Input: part model. Units: mm. Frame: model coordinates. Coordinates: 2 decimals unless noted, no trailing zeros. Loops run counter-clockwise (first coordinate to the right, second up) from the corner with the lowest first, then second, coordinate; pieces in that order, holes last. Notation, with made-up numbers: M -14,47 L 2,47 A10 ccw 2,55 Z; hole C 1.25,61 d10. An arc over 180 degrees is marked long. Use a Markdown table: item, result. Add a question column.
1. Section C-C on y = 2.25. Output: boundary loops of the cut face in (x, z), then the cut area to 3 significant figures.
2. Line query: L1, parallel to Y at x = 1, z = -2; L2, parallel to Z at x = 4.5, y = -1; L3, parallel to Z at x = 2.25, y = -2. Output: solid intervals per line, ascending. Write a range as [from, to].
3. Section B-B on x = 2.5. Output: boundary loops of the cut face in (y, z) (3 decimals), then the cut area to 3 significant figures.
4. Section A-A on z = 12. Output: boundary loops of the cut face in (x, y), then the cut area to 3 significant figures.
5. Pin query (flat end, axial travel): pin 1 (2 mm diameter, centred on x = 0.5, y = -4.5, fed in from +Z); pin 2 (1.8 mm diameter, centred on y = 0, z = -12, fed in from -X); pin 3 (0.7 mm diameter, centred on y = 0, z = 15, fed in from +X); pin 4 (2 mm diameter, centred on x = 5.5, y = 3, fed in from -Z). Return the tip coordinate at first contact, or that it passes through.
6. Section D-D on y = 6.5. Output: boundary loops of the cut face in (x, z).
7. Draft query along Y for faces 1 (the cylindrical face through (3.131, -0.119, -14.463)), 2 (the flat face through (3, -8, 0)), 3 (the cylindrical face through (3, 0, -26)), 4 (the flat face through (6.35, 3.4, 0.4)). Return one class per face: +Y half, -Y half, draft (parallel to the pull), parting line (faces both ways), or undercut.
Autodesk Inventor part; units mm, degrees
ref_plane "YZ Plane" through (0, 0, 0) normal (1, 0, 0) x (0, 1, 0)
ref_plane "XZ Plane" through (0, 0, 0) normal (0, 1, 0) x (-1, 0, 0)
ref_plane "XY Plane" through (0, 0, 0) normal (0, 0, 1) x (1, 0, 0)
sketch "Block1" plane through (0, 0, 0) normal (0, 0, 1) x (1, 0, 0)
  circle A0 centre (-34.5082, -40.3774) radius 0.55
  circle A1 centre (-31.5082, -40.3774) radius 0.55
  circle A2 centre (-28.5082, -40.3774) radius 0.55
  point P0 (-31.5082, -40.3774)
  dimension "d7" = 1.1
  dimension "d8" = 1.1
  dimension "d9" = 1.1
sketch "Sketch1" plane through (0, 0, 0) normal (1, 0, 0) x (0, 1, 0)
  circle A0 centre (0, 0) radius 3.175
  line L0 (8, 0) -> (8, -60)
  line L1 (-8, 0) -> (-8, -60)
  arc A1 (-8, -60) -> (8, -60) centre (0, -60) ccw
  circle A2 centre (0, -60) radius 3.175
  line L2 (0, -105.9654) -> (0, 47.9942) construction
  line L3 (8, 0) -> (-8, 0) construction
  line L4 (8, 0) -> (8, 18)
  line L5 (-8, 0) -> (-8, 18)
  arc A3 (8, 18) -> (-8, 18) centre (0, 18) ccw
  line L6 (-36, 0) -> (58.5, 0) construction
  line L7 (0, -45) -> (-22.5, -83.9711)
  line L8 (0, -45) -> (45, -45) construction
  line L9 (-22.5, -83.9711) -> (-22.5, -45)
  line L10 (-22.5, -45) -> (0, -45)
  line L11 (-22.5, -45) -> (-8, -30)
  circle A4 centre (0, -18) radius 8
  circle A5 centre (0, -12) radius 0.55
  circle A6 centre (0, -15) radius 0.55
  circle A7 centre (0, -18) radius 0.55
  circle A8 centre (0, 12) radius 0.55
  circle A9 centre (0, 15) radius 0.55
  circle A10 centre (0, 18) radius 0.55
  point P0 (0, 0)
  point P1 (-8, -58.8564)
  point P2 (-8, -18)
  point P3 (8, -18)
  dimension "d0" = 6.35
  dimension "d2" = 16
  dimension "d4" = 6.35
  dimension "d11" = 12
  dimension "d12" = 60
  dimension "d13" = 45
  dimension "d14" = 120
  dimension "d15" = 45
extrude "Extrusion2" add sketch "Sketch1" along normal blind 6.35 contours L0 A4 L1 L5 A3 L4 | A4
equation "\"d7\" = d9"
equation "\"d8\" = d9"
properties part number "Spacer Skiba"
Answers below:
| question | item | result |
|---|---|---|
| 1 | outline | M 0,-25.68 L 6.35,-25.68 L 6.35,-2.24 L 0,-2.24 Z; M 0,2.24 L 6.35,2.24 L 6.35,25.68 L 0,25.68 Z |
| 1 | area | 298 mm² |
| 2 | L1 | y = [-8, -2.47], [2.47, 8] |
| 2 | L2 | z = [-25.94, -3.01], [3.01, 25.94] |
| 2 | L3 | z = [-25.75, -2.47], [2.47, 25.75] |
| 3 | outline | M -8,-18 A8 ccw 8,-18 L 8,18 A8 ccw -8,18 Z; hole C 0,0 d6.35; hole C 0,-18 d1.1; hole C 0,-15 d1.1; hole C 0,-12 d1.1; hole C 0,12 d1.1; hole C 0,15 d1.1; hole C 0,18 d1.1 |
| 3 | area | 740 mm² |
| 4 | outline | M 0,-8 L 6.35,-8 L 6.35,-0.55 L 0,-0.55 Z; M 0,0.55 L 6.35,0.55 L 6.35,8 L 0,8 Z |
| 4 | area | 94.6 mm² |
| 5 | pin 1 | stops at z = 25.19 |
| 5 | pin 2 | stops at x = 0 |
| 5 | pin 3 | passes through |
| 5 | pin 4 | stops at z = -25.75 |
| 6 | outline | M 0,-22.66 L 6.35,-22.66 L 6.35,22.66 L 0,22.66 Z |
| 7 | face 1 | undercut |
| 7 | face 2 | -Y half |
| 7 | face 3 | parting line |
| 7 | face 4 | draft |
